```python
from build123d import *

# Parameters (mm, degrees)
SKETCH_2_R          = 13.25
CUT_EXTRUDE_1_DEPTH = 36.215875749


with BuildPart() as part:
    # 草图1 → 旋转1 (revolve)
    with BuildSketch(Plane.XY, mode=Mode.PRIVATE) as revolve_1_sk:
        Polygon((11.881076893, 20.979940533), (18, 20.979940533), (18, 19.979940533), (14.25, 19.979940533), (14.25, 14.979940533), (20, 14.979940533), (20, 13.979940533), (14.25, 13.979940533), (14.25, 6.979940533), (20, 6.979940533), (20, 5.979940533), (14.25, 5.979940533), (14.25, 0.979940533), (18, 0.979940533), (18, 0), (4.648229123, 0), (0, 0), (0, 20.979940533), align=None)
    revolve(revolve_1_sk.sketch.rotate(Axis((0, 0, 0), (0, 1, 0)), 90), axis=Axis((0, 0, 0), (0, 1, 0)))

    # 草图2 → 切除-拉伸1 (cut, through all)
    with BuildSketch(Plane(origin=(0, 20.979940533, 0), x_dir=(1, 0, 0), z_dir=(0, 1, 0))):
        with Locations(Location((0, 0, 0), (0, 0, 270))):
            Circle(SKETCH_2_R)
    extrude(amount=-CUT_EXTRUDE_1_DEPTH, mode=Mode.SUBTRACT)


solid = part.part
```
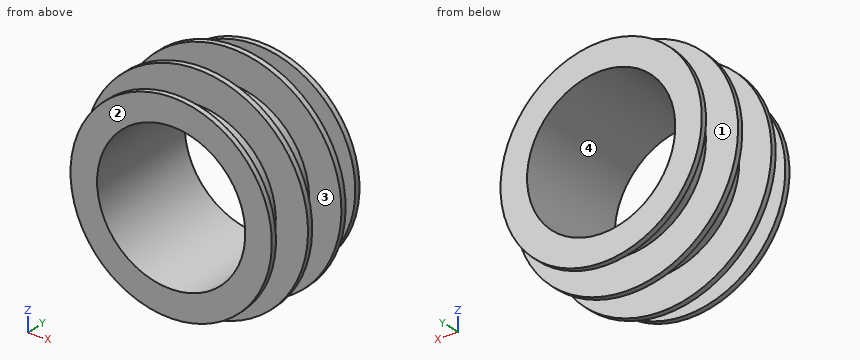
Input: part model. Units: mm. Frame: model coordinates. Face numbers are marked on the shaded views. A direction names the side the tool comes from. Give positions to 0.01 mm unless a question says otherwise; leave off trailing zeros. Loops run counter-clockwise (first coordinate to the right, second up) from the corner with the lowest first, then second, coordinate; pieces in that order, holes last. Notation, with made-up numbers: (-4, 81) -> (54, 81) arc R23 cw to (54, 101) -> close; hole circle Ø9 at (0.25, 56.5). An arc over 180 degrees is marked (long way). Use a Markdown table: item, result.
Q1. Section query C-C, the plane y = 12.5. Return the cut outline in (x, z), plus the area to 3 significant figures.
Entries:
| item | result |
|---|---|
| outline | circle Ø28.5 at (0, 0); hole circle Ø26.5 at (0, 0) |
| area | 86.4 mm² |
Q2. First-contact query: P1, Ø11, axis at x = -5, z = 5, coming from the +Y side; P2, Ø3, axis at x = 8.5, y = 17.5, coming from the +Z side; P3, Ø1.5, axis at y = 13.5, z = 9, coming from the -X side; P4, Ø3, axis at x = 7, y = 15.5, coming from the -Z side. Flat tips, straight axial feed; report the tip coordinate or a pass-through.
Entries:
| item | result |
|---|---|
| P1 | passes through |
| P2 | stops at z = 12.41 |
| P3 | stops at x = -18.14 |
| P4 | stops at z = -19.2 |
Q3. Pull-direction query (Z, two-part tool) for the marked faces 3 and 4; classes: pulls with the +Z half, pulls with the -Z half, needs draft (parallel to the pull), parting line crosses it, or undercut.
Entries:
| item | result |
|---|---|
| face 3 | needs draft |
| face 4 | undercut |
Q4. Access query for the marked faces 1 and 2. Directions: +Z, -Z, +X, -X, +Y, -Y. A direction counts if a zero-diameter tool reaches every point of the face in a straight line with its end or side. Return the directions, or none.
Entries:
| item | result |
|---|---|
| face 1 | none |
| face 2 | +Z, -Z, +X, -X, -Y |
Q5. Ray query, probe 1 along Y at (x, z) = (15.5, -7); probe 2 along Y at (x, z) = (10, 17); probe 3 along X at (y, z) = (8, 0). Return the intervals inside material, ascending. Write a range as from..to.
Entries:
| item | result |
|---|---|
| probe 1 | y = 0..0.98, 5.98..6.98, 13.98..14.98, 19.98..20.98 |
| probe 2 | y = 5.98..6.98, 13.98..14.98 |
| probe 3 | x = -14.25..-13.25, 13.25..14.25 |
